The listing builds one solid part. Answer for the finished solid, in the listing's coordinates (mm). A direction names the side the tool comes from. Give positions to 0.01 mm unless a question says otherwise; leave off trailing zeros. Write each loop counter-clockwise with the first axis right and the second up, starting at its lowest first coordinate (ties: lowest second). Pieces come first, ordered by that corner, then holes. Notation, with made-up numbers: (56.25, 25.25) -> (106.25, 25.25) arc R20 cw to (106.25, 45.25) -> close; hole circle Ø1 at (57.5, 16). An arc over 180 degrees is marked (long way). Put each result on its own line as item: value. Start each with the question number.
1) Find the intervals of material crossed by line 1 along X through (y, z) = (0.7, 0); line 2 along Z through (x, y) = (6, 2); line 3 along Z through (x, y) = (16.5, 2.1), in increasing order. Write a range as from..to.
2) A cutting plane is placed at C-C (y = 0.8). Write down the section's boundary in (x, z).
3) A cutting plane is placed at D-D (x = -15.5). Write down the section's boundary in (y, z).
4) For a pull along Z with two mould halves and no side action, classify faces 1 (the flat face through (-20, 2, -19)), 2 (the flat face through (1, 0, 8)), 3 (the flat face through (0, 2, -20.803)), 4 (the cylindrical face through (-39.05, 1.48, -8.67)) as released by +Z, released by -Z, zero draft, split by the parting line, or undercut.
5) A cutting plane is placed at A-A (x = 0). Write down the section's boundary in (y, z), then the cut area to 3 significant figures.
6) For faces 5 (the flat face through (20, 2, -19)), 6 (the flat face through (1, 3, 8)), determine the directions among +Z, -Z, +X, -X, +Y, -Y from which every point of the face is accessible in a straight line to the end or side of a thin tool.
7) Flat-ended cylindrical pins translate along their axes: pin 1 Ø1.5 at (y, z) = (2, -19.5) entering from +X; pin 2 Ø1.5 at (x, y) = (26.5, 2) entering from +Z; pin 3 Ø1.5 at (x, y) = (-5, 1.5) entering from -Z; pin 4 Ø3 at (x, z) = (29.5, 30.5) entering from -Y. Find the tip coordinate at first contact, or state that the pin passes through.
8) A cutting plane is placed at B-B (z = 0). Write down the section's boundary in (x, y), then the cut area to 3 significant figures.
from build123d import *

# Parameters (mm, degrees)
SKETCH1_R           = 40
BOSS_EXTRUDE1_DEPTH = 3
SKETCH2_R           = 1
CUT_EXTRUDE1_DEPTH  = 3
SKETCH3_W           = 40
SKETCH3_H           = 3
CUT_EXTRUDE2_DEPTH  = 10


with BuildPart() as part:
    # Sketch1 → Boss-Extrude1 (new body)
    with BuildSketch(Plane(origin=(0, 0, 0), x_dir=(1, 0, 0), z_dir=(0, 1, 0))):
        with Locations(Location((0, 0, 0), (0, 0, 270))):
            Circle(SKETCH1_R)
    extrude(amount=BOSS_EXTRUDE1_DEPTH)

    # Sketch2 → Cut-Extrude1 (cut)
    with BuildSketch(Plane(origin=(0, 3, 0), x_dir=(1, 0, 0), z_dir=(0, 1, 0))):
        with Locations(Location((0, 0, 0), (0, 0, 270))):
            Circle(SKETCH2_R)
    extrude(amount=-CUT_EXTRUDE1_DEPTH, mode=Mode.SUBTRACT)

    # Sketch3 → Cut-Extrude2 (cut)
    with BuildSketch(Plane(origin=(0, 3, 0), x_dir=(1, 0, 0), z_dir=(0, 1, 0))):
        with Locations((0, 19.302837328)):
            Rectangle(SKETCH3_W, SKETCH3_H)
    extrude(amount=-CUT_EXTRUDE2_DEPTH, mode=Mode.SUBTRACT)


solid = part.part
Reply:
1. line 1: x = -40..-1, 1..40
1. line 2: z = -39.55..-20.8, -17.8..39.55
1. line 3: z = -36.44..-20.8, -17.8..36.44
2. outline: circle Ø80 at (0, 0); hole (-20, -20.8) -> (20, -20.8) -> (20, -17.8) -> (-20, -17.8) -> close; hole circle Ø2 at (0, 0)
3. outline: (0, -36.87) -> (3, -36.87) -> (3, -20.8) -> (0, -20.8) -> close; (0, -17.8) -> (3, -17.8) -> (3, 36.87) -> (0, 36.87) -> close
4. face 1: undercut
4. face 2: zero draft
4. face 3: undercut
4. face 4: split by the parting line
5. outline: (0, -40) -> (3, -40) -> (3, -20.8) -> (0, -20.8) -> close; (0, -17.8) -> (3, -17.8) -> (3, -1) -> (0, -1) -> close; (0, 1) -> (3, 1) -> (3, 40) -> (0, 40) -> close
5. area: 225 mm2
6. face 5: +Y, -Y
6. face 6: +Z, -Z, +X, -X, +Y
7. pin 1: stops at x = 35.33
7. pin 2: stops at z = 30.61
7. pin 3: stops at z = -39.77
7. pin 4: passes through
8. outline: (-40, 0) -> (-1, 0) -> (-1, 3) -> (-40, 3) -> close; (1, 0) -> (40, 0) -> (40, 3) -> (1, 3) -> close
8. area: 234 mm2
